Here's the drawing with two shaded views (mm, measured from the low corner). I have some questions. Give positions to 0.01 mm unless a question says otherwise; leave off trailing zeros. Write each loop counter-clockwise with the first axis right and the second up, starting at its lowest first coordinate (ties: lowest second). Pieces come first, ordered by that corner, then holes.
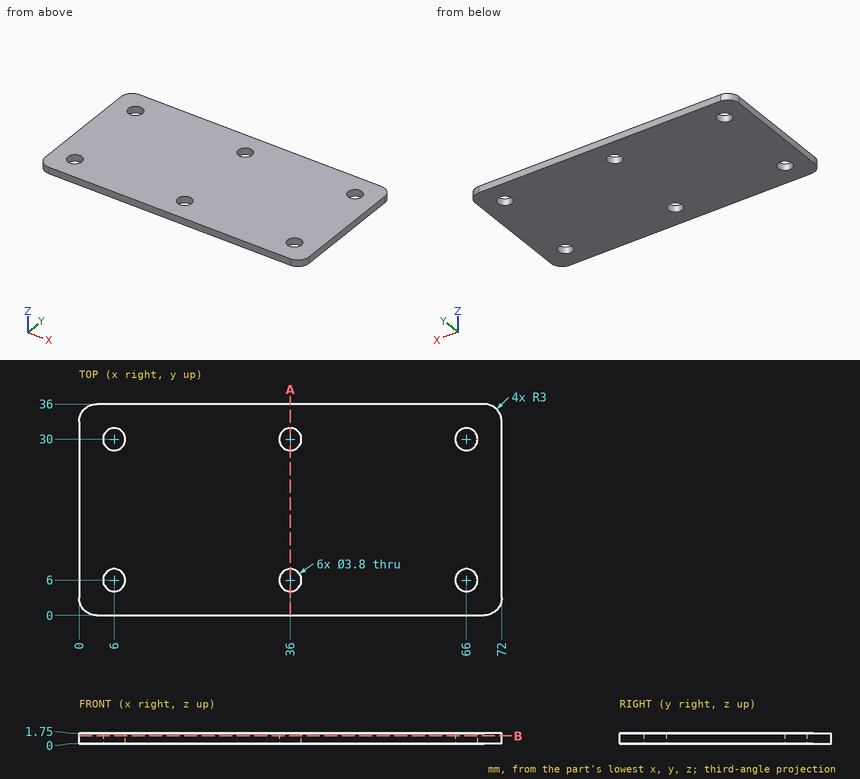
1) Please list where these lines run through material, in increasing order: L1, parallel to Y at x = 6, z = 0.7; L2, parallel to Y at x = 65, z = 0.8; L3, parallel to X at y = 34, z = 1.4.
Values follow:
L1: y = 0 to 4.1, 7.9 to 28.1, 31.9 to 36
L2: y = 0 to 4.38, 7.62 to 28.38, 31.62 to 36
L3: x = 0.17 to 71.83
2) For pin 1 Ø2.5 at (x, y) = (36, 6) entering from +Z, with a flat end and sliding along its axis, tell me the tip position at first contact or that it passes through.
Values follow:
pin 1: passes through
3) Suppose I cut it at B-B on z = 1.3. Write out the boundary of the cut face in (x, y), plus the area to 3 significant figures.
Values follow:
outline: (0, 3) arc R3 ccw to (3, 0) - (69, 0) arc R3 ccw to (72, 3) - (72, 33) arc R3 ccw to (69, 36) - (3, 36) arc R3 ccw to (0, 33) - close; hole circle Ø3.8 at (6, 6); hole circle Ø3.8 at (6, 30); hole circle Ø3.8 at (36, 6); hole circle Ø3.8 at (36, 30); hole circle Ø3.8 at (66, 6); hole circle Ø3.8 at (66, 30)
area: 2,520 mm2
4) Suppose I cut it at A-A on x = 36. Write out the boundary of the cut face in (y, z).
Values follow:
outline: (0, 0) - (4.1, 0) - (4.1, 1.75) - (0, 1.75) - close; (7.9, 0) - (28.1, 0) - (28.1, 1.75) - (7.9, 1.75) - close; (31.9, 0) - (36, 0) - (36, 1.75) - (31.9, 1.75) - close
